from build123d import *

# Parameters (mm, degrees)
SKETCH_1_W          = 89
SKETCH_1_H          = 134
EXTRUDE_2_DEPTH     = 16.5
SKETCH_4_W          = 75
SKETCH_4_H          = 120
CUT_EXTRUDE_1_DEPTH = 28
CUT_EXTRUDE1_REACH  = 88.938
SKETCH4_R           = 1.5
CUT_EXTRUDE2_REACH  = 144.157
SKETCH7_W           = 13.210021701
SKETCH7_H           = 6.5
SKETCH7_W_2         = 36.926143907
SKETCH7_H_2         = 11.2004
CUT_EXTRUDE3_REACH  = 114.615
SKETCH8_R           = 2.5
FILLET3_R           = 1
SKETCH9_R           = 1.6
CUT_EXTRUDE4_DEPTH  = 87.938196439
CUT_EXTRUDE5_DEPTH  = 2.5


with BuildPart() as part:
    # 草圖1 → 填料-伸長2 (new, symmetric)
    with BuildSketch(Plane(origin=(0, 0, 0), x_dir=(1, 0, 0), z_dir=(0, 1, 0))):
        Rectangle(SKETCH_1_W, SKETCH_1_H)
    extrude(amount=EXTRUDE_2_DEPTH, both=True)

    # 草圖4 → 除料-伸長1 (cut)
    with BuildSketch(Plane(origin=(0, 16.5, 0), x_dir=(1, 0, 0), z_dir=(0, 1, 0))):
        Rectangle(SKETCH_4_W, SKETCH_4_H)
    extrude(amount=-CUT_EXTRUDE_1_DEPTH, mode=Mode.SUBTRACT)

    # Sketch4 → Cut-Extrude1 (cut, up to next)
    with BuildSketch(Plane.XZ.offset(16.5), mode=Mode.PRIVATE) as cut_extrude1_sk1:
        with Locations(Location((-32.8808, -9.5, 0), (0, 0, 270))):
            Circle(SKETCH4_R)
    cut_extrude1_tool1 = extrude(cut_extrude1_sk1.sketch, amount=-CUT_EXTRUDE1_REACH, mode=Mode.PRIVATE) & part.part
    # Sketch4 → Cut-Extrude1 (cut, up to next)
    with BuildSketch(Plane.XZ.offset(16.5), mode=Mode.PRIVATE) as cut_extrude1_sk2:
        with Locations(Location((-8.3808, -9.5, 0), (0, 0, 270))):
            Circle(SKETCH4_R)
    cut_extrude1_tool2 = extrude(cut_extrude1_sk2.sketch, amount=-CUT_EXTRUDE1_REACH, mode=Mode.PRIVATE) & part.part
    # Sketch4 → Cut-Extrude1 (cut, up to next)
    with BuildSketch(Plane.XZ.offset(16.5), mode=Mode.PRIVATE) as cut_extrude1_sk3:
        with Locations(Location((-32.8808, -56, 0), (0, 0, 270))):
            Circle(SKETCH4_R)
    cut_extrude1_tool3 = extrude(cut_extrude1_sk3.sketch, amount=-CUT_EXTRUDE1_REACH, mode=Mode.PRIVATE) & part.part
    # Sketch4 → Cut-Extrude1 (cut, up to next)
    with BuildSketch(Plane.XZ.offset(16.5), mode=Mode.PRIVATE) as cut_extrude1_sk4:
        with Locations(Location((-8.3808, -56, 0), (0, 0, 270))):
            Circle(SKETCH4_R)
    cut_extrude1_tool4 = extrude(cut_extrude1_sk4.sketch, amount=-CUT_EXTRUDE1_REACH, mode=Mode.PRIVATE) & part.part
    # Sketch4 → Cut-Extrude1 (cut, up to next)
    with BuildSketch(Plane.XZ.offset(16.5), mode=Mode.PRIVATE) as cut_extrude1_sk5:
        with Locations(Location((1.5402, -10.375, 0), (0, 0, 270))):
            Circle(SKETCH4_R)
    cut_extrude1_tool5 = extrude(cut_extrude1_sk5.sketch, amount=-CUT_EXTRUDE1_REACH, mode=Mode.PRIVATE) & part.part
    # Sketch4 → Cut-Extrude1 (cut, up to next)
    with BuildSketch(Plane.XZ.offset(16.5), mode=Mode.PRIVATE) as cut_extrude1_sk6:
        with Locations(Location((32.579, -10.375, 0), (0, 0, 270))):
            Circle(SKETCH4_R)
    cut_extrude1_tool6 = extrude(cut_extrude1_sk6.sketch, amount=-CUT_EXTRUDE1_REACH, mode=Mode.PRIVATE) & part.part
    # Sketch4 → Cut-Extrude1 (cut, up to next)
    with BuildSketch(Plane.XZ.offset(16.5), mode=Mode.PRIVATE) as cut_extrude1_sk7:
        with Locations(Location((1.5402, -55.079, 0), (0, 0, 270))):
            Circle(SKETCH4_R)
    cut_extrude1_tool7 = extrude(cut_extrude1_sk7.sketch, amount=-CUT_EXTRUDE1_REACH, mode=Mode.PRIVATE) & part.part
    # Sketch4 → Cut-Extrude1 (cut, up to next)
    with BuildSketch(Plane.XZ.offset(16.5), mode=Mode.PRIVATE) as cut_extrude1_sk8:
        with Locations(Location((32.579, -55.079, 0), (0, 0, 270))):
            Circle(SKETCH4_R)
    cut_extrude1_tool8 = extrude(cut_extrude1_sk8.sketch, amount=-CUT_EXTRUDE1_REACH, mode=Mode.PRIVATE) & part.part
    add(cut_extrude1_tool1.solids().sort_by_distance((-32.8808, -16.5, -9.5))[0], mode=Mode.SUBTRACT)
    add(cut_extrude1_tool2.solids().sort_by_distance((-8.3808, -16.5, -9.5))[0], mode=Mode.SUBTRACT)
    add(cut_extrude1_tool3.solids().sort_by_distance((-32.8808, -16.5, -56))[0], mode=Mode.SUBTRACT)
    add(cut_extrude1_tool4.solids().sort_by_distance((-8.3808, -16.5, -56))[0], mode=Mode.SUBTRACT)
    add(cut_extrude1_tool5.solids().sort_by_distance((1.5402, -16.5, -10.375))[0], mode=Mode.SUBTRACT)
    add(cut_extrude1_tool6.solids().sort_by_distance((32.579, -16.5, -10.375))[0], mode=Mode.SUBTRACT)
    add(cut_extrude1_tool7.solids().sort_by_distance((1.5402, -16.5, -55.079))[0], mode=Mode.SUBTRACT)
    add(cut_extrude1_tool8.solids().sort_by_distance((32.579, -16.5, -55.079))[0], mode=Mode.SUBTRACT)

    # Sketch7 → Cut-Extrude2 (cut, up to next)
    with BuildSketch(Plane(origin=(0, 0, -67), x_dir=(-1, 0, 0), z_dir=(0, 0, -1)), mode=Mode.PRIVATE) as cut_extrude2_sk1:
        with Locations((20.850501077, -8.25)):
            Rectangle(SKETCH7_W, SKETCH7_H)
    cut_extrude2_tool1 = extrude(cut_extrude2_sk1.sketch, amount=-CUT_EXTRUDE2_REACH, mode=Mode.PRIVATE) & part.part
    # Sketch7 → Cut-Extrude2 (cut, up to next)
    with BuildSketch(Plane(origin=(0, 0, -67), x_dir=(-1, 0, 0), z_dir=(0, 0, -1)), mode=Mode.PRIVATE) as cut_extrude2_sk2:
        with Locations((-17.096479408, -1.8998)):
            Rectangle(SKETCH7_W_2, SKETCH7_H_2)
    cut_extrude2_tool2 = extrude(cut_extrude2_sk2.sketch, amount=-CUT_EXTRUDE2_REACH, mode=Mode.PRIVATE) & part.part
    add(cut_extrude2_tool1.solids().sort_by_distance((-20.850501, -8.25, -67))[0], mode=Mode.SUBTRACT)
    add(cut_extrude2_tool2.solids().sort_by_distance((17.096479, -1.8998, -67))[0], mode=Mode.SUBTRACT)

    # Sketch8 → Cut-Extrude3 (cut, up to next)
    with BuildSketch(Plane(origin=(44.5, 0, 0), x_dir=(0, 0, -1), z_dir=(1, 0, 0)), mode=Mode.PRIVATE) as cut_extrude3_sk1:
        with Locations((-8.471, -2.3)):
            Circle(SKETCH8_R)
    cut_extrude3_tool1 = extrude(cut_extrude3_sk1.sketch, amount=-CUT_EXTRUDE3_REACH, mode=Mode.PRIVATE) & part.part
    add(cut_extrude3_tool1.solids().sort_by_distance((44.5, -2.3, 8.471))[0], mode=Mode.SUBTRACT)

    # Fillet3
    fillet3_edges = [part.edges().sort_by_distance(p)[0] for p in [
        (-44.5, 16.5, 0),
        (0, 16.5, 67),
        (44.5, 16.5, 0),
        (0, -16.5, 67),
        (-44.5, -16.5, 0),
        (0, -16.5, -67),
        (44.5, -16.5, 0),
        (-20.850501078, -5, -67),
        (-14.245490227, -8.25, -67),
        (-20.850501078, -11.5, -67),
        (-27.455511928, -8.25, -67),
        (17.096479408, 3.7004, -67),
        (35.559551361, -1.8998, -67),
        (17.096479408, -7.5, -67),
        (-1.366592546, -1.8998, -67),
        (44.5, 0, 67),
        (-44.5, 0, 67),
        (-44.5, 0, -67),
        (44.5, 0, -67),
        (44.5, -2.3, 10.971),
        (0, 16.5, -67),
    ]]
    fillet(fillet3_edges, radius=FILLET3_R)

    # Sketch9 → Cut-Extrude4 (cut, through all)
    with BuildSketch(Plane(origin=(0, 16.5, 0), x_dir=(1, 0, 0), z_dir=(0, 1, 0))):
        with Locations(Location((-40.49479618, 62.99479618, 0), (0, 0, 270))):
            Circle(SKETCH9_R)
        with Locations(Location((40.49479618, 62.99479618, 0), (0, 0, 270))):
            Circle(SKETCH9_R)
        with Locations(Location((40.49479618, -62.99479618, 0), (0, 0, 270))):
            Circle(SKETCH9_R)
        with Locations(Location((-40.49479618, -62.99479618, 0), (0, 0, 270))):
            Circle(SKETCH9_R)
    extrude(amount=-CUT_EXTRUDE4_DEPTH, mode=Mode.SUBTRACT)

    # Sketch10 → Cut-Extrude5 (cut)
    with BuildSketch(Plane.XZ.offset(16.5)):
        Polygon((-40.49479618, 66.170222661), (-43.24479618, 64.58250942), (-43.24479618, 61.40708294), (-40.49479618, 59.819369699), (-37.74479618, 61.40708294), (-37.74479618, 64.58250942), align=None)
        Polygon((37.74479618, 64.58250942), (40.49479618, 66.170222661), (43.24479618, 64.58250942), (43.24479618, 61.40708294), (40.49479618, 59.819369699), (37.74479618, 61.40708294), align=None)
        Polygon((37.74479618, -61.40708294), (37.74479618, -64.58250942), (40.49479618, -66.170222661), (43.24479618, -64.58250942), (43.24479618, -61.40708294), (40.49479618, -59.819369699), align=None)
        Polygon((-37.74479618, -64.58250942), (-40.49479618, -66.170222661), (-43.24479618, -64.58250942), (-43.24479618, -61.40708294), (-40.49479618, -59.819369699), (-37.74479618, -61.40708294), align=None)
    extrude(amount=-CUT_EXTRUDE5_DEPTH, mode=Mode.SUBTRACT)


solid = part.part
Verification items for the finished model (mm, model axes). A direction names the side the tool comes from. Coordinates: 2 decimals unless noted, no trailing zeros. Order: outer loops, then holes, each group sorted by start corner. A loop starts at its lowest first (then second) coordinate and runs counter-clockwise, first axis right, second up. Notation, with made-up numbers: M 35.25,35.25 L 44.25,35.25 A24 ccw 44.25,70.25 Z; hole C -7.5,88.25 d7. An arc over 180 degrees is marked long. One line per item, written item: value. Start each with the question number.
Item 1: Sectioned sample at A-A on x = -24.5. Record the cut outline in (y, z), then the cut area to 3 significant figures.
Item 2: Mould release check, pull along X, two halves, no side actions. Record for faces 4 (the flat face through (-10, 0, -67)), 5 (the flat face through (-21, -5, -63)), 6 (the flat face through (44.5, 0, 1)): pulls with the +X half, pulls with the -X half, needs draft (parallel to the pull), parting line crosses it, or undercut.
Item 3: Thickness scan on probe 1 along Z at (x, y) = (1, 8); probe 2 along X at (y, z) = (-2, -8.5); probe 3 along Z at (x, y) = (-39.5, 6.5). Record the ranges inside material, lowest first.
Item 4: Depth check by flat-ended pin: P1, Ø4, axis at x = -40.49, z = 62.99, coming from the -Y side; P2, Ø2, axis at x = 17, y = 3, coming from the -Z side; P3, Ø2.5, axis at x = 32.579, z = -55.079, coming from the +Y side; P4, Ø2, axis at x = 7.5, z = 3, coming from the +Y side. Enter the tip coordinate at first touch or a pass-through.
Item 5: Sectioned sample at C-C on z = 15.5. Record the cut outline in (x, y).
Item 6: Sectioned sample at B-B on y = -2.3. Record the cut outline in (x, z), then the cut area to 3 significant figures.
Item 7: Access from +Z, -Z, +X, -X, +Y, -Y to the whole of each face (thin tool, end or side, straight path). Record for faces 1 (the flat face through (-1, -16.5, -1)), 2 (the flat face through (-14.245, -8, -63)), 3 (the flat face through (-39, -14, -64)).
Item 8: Sectioned sample at D-D on x = 19. Record the cut outline in (y, z), then the cut area to 3 significant figures.
Calculated:
1. outline: M -16.5,-66 A1 ccw -15.5,-67 L -12.5,-67 A1 ccw -11.5,-66 L -11.5,60 L 16.5,60 L 16.5,66 A1 ccw 15.5,67 L -15.5,67 A1 ccw -16.5,66 Z; M -5,-66 A1 ccw -4,-67 L 15.5,-67 A1 ccw 16.5,-66 L 16.5,-60 L -5,-60 Z
1. area: 1,020 mm^2
2. face 4: needs draft
2. face 5: undercut
2. face 6: pulls with the +X half
3. probe 1: -67 to -60, 60 to 67
3. probe 2: -44.5 to -37.5, 37.5 to 44.5
3. probe 3: -67 to -64.25, -61.74 to 61.74, 64.25 to 67
4. P1: y = -14
4. P2: z = -66.71
4. P3: through
4. P4: y = -11.5
5. outline: M -44.5,-15.5 A1 ccw -43.5,-16.5 L 43.5,-16.5 A1 ccw 44.5,-15.5 L 44.5,15.5 A1 ccw 43.5,16.5 L 37.5,16.5 L 37.5,-11.5 L -37.5,-11.5 L -37.5,16.5 L -43.5,16.5 A1 ccw -44.5,15.5 Z
6. outline: M -44.5,-66 A1 ccw -43.5,-67 L -2.37,-67 A1 ccw -1.37,-66 L -1.37,-60 L -37.5,-60 L -37.5,60 L 37.5,60 L 37.5,10.97 L 43.5,10.97 A1 ccw 44.5,11.97 L 44.5,66 A1 ccw 43.5,67 L -43.5,67 A1 ccw -44.5,66 Z; M 35.56,-66 A1 ccw 36.56,-67 L 43.5,-67 A1 ccw 44.5,-66 L 44.5,4.97 A1 ccw 43.5,5.97 L 37.5,5.97 L 37.5,-60 L 35.56,-60 Z; hole C -40.49,-62.99 d3.2; hole C -40.49,62.99 d3.2; hole C 40.49,-62.99 d3.2; hole C 40.49,62.99 d3.2
6. area: 2,600 mm^2
7. face 1: +Z, -Z, +X, -X, -Y
7. face 2: -Z
7. face 3: -Y
8. outline: M -16.5,-66 A1 ccw -15.5,-67 L -8.5,-67 A1 ccw -7.5,-66 L -7.5,-60 L -11.5,-60 L -11.5,60 L 16.5,60 L 16.5,66 A1 ccw 15.5,67 L -15.5,67 A1 ccw -16.5,66 Z; M 3.7,-66 A1 ccw 4.7,-67 L 15.5,-67 A1 ccw 16.5,-66 L 16.5,-60 L 3.7,-60 Z
8. area: 982 mm^2
